Part model, mm, in its own coordinate system. A direction names the side the tool comes from. Round coordinates to 2 decimals unless told otherwise and drop trailing zeros. Loops run counter-clockwise (first coordinate to the right, second up) from the corner with the lowest first, then second, coordinate; pieces in that order, holes last.
1) Mould opens along X. For faces 5 (the flat face through (150, -55, -456)), 6 (the flat face through (69, -70, -900)), 7 (the flat face through (67.5, -183, -861)), 8 (the cylindrical face through (73.698, -339.915, -75.07)) say: +X half, -X half, draft (parallel to the pull), parting line (faces both ways), or undercut.
2) Probe line 1 (Y direction, x = 75, z = -825.75); line 2 (Z direction, x = 110, y = -300); line 3 (Y direction, x = 136.5, z = -633). List the from-to ranges inside material, lowest first.
3) Band-saw the part on D-D, the plane y = -265. Write the cut outline in (x, z), then the cut area to 4 significant figures.
4) Band-saw the part on C-C, the plane y = -220.5. Write the cut outline in (x, z), then the cut area to 3 significant figures.
5) Band-saw the part on A-A, the plane y = -330. Write the cut outline in (x, z) (3 decimals).
6) Band-saw the part on B-B, the plane z = -750. Write the cut outline in (x, y).
7) 3-axis set-ups, long thin cutter, end or side, ignore diameter. For faces 1 (the flat face through (76, -183, -820)), 2 (the flat face through (47, -47, -444)), 3 (the cylindrical face through (65, -330, -825)), 4 (the flat face through (82.5, -213, -40)): which of +Z, -Z, +X, -X, +Y, -Y reach the whole face in a straight line?
8) Drop flat-ended pins along their axis: P1, Ø6, axis at x = 73, y = -326, coming from the +Z side; P2, Ø1, axis at x = 47.5, y = -99.5, coming from the -Z side; P3, Ø1, axis at x = 127, z = -653.5, coming from the -Y side. Give the stop position or say it passes through.
from build123d import *

# Parameters (mm, degrees)
F0_W      = 150
F0_H      = 900
F1_DEPTH  = 80
F2_W      = 15
F2_H      = 65
F3_DEPTH  = 270
F5_DEPTH  = 25
F7_DEPTH  = 25
F9_DEPTH  = 25
F11_DEPTH = 25
F13_DEPTH = 25
F15_DEPTH = 25
F16_R     = 10
F17_DEPTH = 10
F18_R     = 10
F19_DEPTH = 10
F21_DEPTH = 900.001


with BuildPart() as f1:
    # F0 (on Front) → F1 (new body)
    with BuildSketch(Plane.XZ):
        with Locations((75, -450)):
            Rectangle(F0_W, F0_H)
    extrude(amount=F1_DEPTH)

    # F2 (on face) → F3 (join)
    with BuildSketch(Plane.XZ.offset(80)):
        Polygon((67.5, -65), (0, -65), (0, -80), (150, -80), (150, -65), (82.5, -65), align=None)
        with Locations((75, -32.5)):
            Rectangle(F2_W, F2_H)
        Polygon((150, -820), (0, -820), (0, -835), (67.5, -835), (82.5, -835), (150, -835), align=None)
        with Locations((75, -867.5)):
            Rectangle(F2_W, F2_H)
    extrude(amount=F3_DEPTH)

    # F4 (on face) → F5 (cut)
    with BuildSketch(Plane(origin=(67.5, 0, 0), x_dir=(0, -1, 0), z_dir=(-1, 0, 0))):
        Polygon((350, 0), (150, 0), (350, -32.5), align=None)
    extrude(amount=-F5_DEPTH, mode=Mode.SUBTRACT)

    # F6 (on face) → F7 (cut)
    with BuildSketch(Plane.XY.offset(-65)):
        Polygon((150, -150), (116.25, -350), (150, -350), align=None)
    extrude(amount=-F7_DEPTH, mode=Mode.SUBTRACT)

    # F8 (on face) → F9 (cut)
    with BuildSketch(Plane.XY.offset(-65)):
        Polygon((0, -350), (33.75, -350), (0, -150), align=None)
    extrude(amount=-F9_DEPTH, mode=Mode.SUBTRACT)

    # F10 (on face) → F11 (cut)
    with BuildSketch(Plane(origin=(0, 0, -835), x_dir=(1, 0, 0), z_dir=(0, 0, -1))):
        Polygon((150, 350), (116.25, 350), (150, 150), align=None)
    extrude(amount=-F11_DEPTH, mode=Mode.SUBTRACT)

    # F12 (on face) → F13 (cut)
    with BuildSketch(Plane(origin=(0, 0, -835), x_dir=(1, 0, 0), z_dir=(0, 0, -1))):
        Polygon((0, 150), (33.75, 350), (0, 350), align=None)
    extrude(amount=-F13_DEPTH, mode=Mode.SUBTRACT)

    # F14 (on face) → F15 (cut)
    with BuildSketch(Plane(origin=(67.5, 0, 0), x_dir=(0, -1, 0), z_dir=(-1, 0, 0))):
        Polygon((350, -900), (350, -867.5), (150, -900), align=None)
    extrude(amount=-F15_DEPTH, mode=Mode.SUBTRACT)

    # F16 (on face) → F17 (cut)
    with BuildSketch(Plane(origin=(0, 0, -80), x_dir=(1, 0, 0), z_dir=(0, 0, -1))):
        with Locations((75, 330)):
            Circle(F16_R)
    extrude(amount=-F17_DEPTH, mode=Mode.SUBTRACT)

    # F18 (on face) → F19 (cut)
    with BuildSketch(Plane.XY.offset(-820)):
        with Locations((75, -330)):
            Circle(F18_R)
    extrude(amount=-F19_DEPTH, mode=Mode.SUBTRACT)

    # F20 (on face) → F21 (cut, through all)
    with BuildSketch(Plane.XY):
        Polygon((130, -20), (20, -20), (75, -75), align=None)
        Polygon((150, 0), (0, 0), (20, -20), (130, -20), align=None)
        Polygon((20, -20), (0, 0), (0, -20), align=None)
        Polygon((150, -20), (150, 0), (130, -20), align=None)
    extrude(amount=-F21_DEPTH, mode=Mode.SUBTRACT)


solid = f1.part
Reported:
1. face 5: +X half
1. face 6: draft
1. face 7: -X half
1. face 8: undercut
2. line 1: y = -350 to -340, -320 to -75
2. line 2: z = -835 to -820, -80 to -65
2. line 3: y = -80 to -20
3. outline: (19.41, -835) - (67.5, -835) - (67.5, -881.31) - (82.5, -881.31) - (82.5, -835) - (130.59, -835) - (130.59, -820) - (19.41, -820) - close; (19.41, -80) - (130.59, -80) - (130.59, -65) - (82.5, -65) - (82.5, -18.69) - (67.5, -18.69) - (67.5, -65) - (19.41, -65) - close
3. area: 4,725 mm2
4. outline: (11.9, -835) - (67.5, -835) - (67.5, -888.54) - (82.5, -888.54) - (82.5, -835) - (138.1, -835) - (138.1, -820) - (11.9, -820) - close; (11.9, -80) - (138.1, -80) - (138.1, -65) - (82.5, -65) - (82.5, -11.46) - (67.5, -11.46) - (67.5, -65) - (11.9, -65) - close
4. area: 5,390 mm2
5. outline: (30.375, -835) - (67.5, -835) - (67.5, -870.75) - (82.5, -870.75) - (82.5, -835) - (119.625, -835) - (119.625, -820) - (85, -820) - (85, -830) - (65, -830) - (65, -820) - (30.375, -820) - close; (30.375, -80) - (65, -80) - (65, -70) - (85, -70) - (85, -80) - (119.625, -80) - (119.625, -65) - (82.5, -65) - (82.5, -29.25) - (67.5, -29.25) - (67.5, -65) - (30.375, -65) - close
6. outline: (0, -80) - (150, -80) - (150, -20) - (130, -20) - (75, -75) - (20, -20) - (0, -20) - close
7. face 1: +X, -X, -Y
7. face 2: +Z, -Z, +Y
7. face 3: none
7. face 4: +Z, +X, -Y
8. P1: stops at z = -28.11
8. P2: stops at z = -835
8. P3: stops at y = -80
